from build123d import *

# Parameters (mm, degrees)
CROQUIS2_W              = 500
CROQUIS2_H              = 350
SALIENTE_EXTRUIR1_DEPTH = 50
CROQUIS3_W              = 125
CROQUIS3_H              = 87.5
SALIENTE_EXTRUIR2_DEPTH = 500


with BuildPart() as part:
    # Croquis2 → Saliente-Extruir1 (new body)
    with BuildSketch(Plane(origin=(0, 0, 0), x_dir=(1, 0, 0), z_dir=(0, 1, 0))):
        Rectangle(CROQUIS2_W, CROQUIS2_H)
    extrude(amount=SALIENTE_EXTRUIR1_DEPTH)

    # Croquis3 → Saliente-Extruir2 (add)
    with BuildSketch(Plane.XZ):
        with Locations((-187.5, 131.25)):
            Rectangle(CROQUIS3_W, CROQUIS3_H)
        with Locations((-187.5, -131.25)):
            Rectangle(CROQUIS3_W, CROQUIS3_H)
        with Locations((187.5, -131.25)):
            Rectangle(CROQUIS3_W, CROQUIS3_H)
        with Locations((187.5, 131.25)):
            Rectangle(CROQUIS3_W, CROQUIS3_H)
    extrude(amount=SALIENTE_EXTRUIR2_DEPTH)


solid = part.part
Could you check a few things on this model? Use its own coordinates, in mm. A direction names the side the tool comes from. Round coordinates to 2 decimals unless told otherwise and drop trailing zeros. Write each loop counter-clockwise with the first axis right and the second up, starting at its lowest first coordinate (ties: lowest second). Pieces come first, ordered by that corner, then holes. Notation, with made-up numbers: (81.5, 75.25) - (104.5, 75.25) arc R18 cw to (104.5, 91.25) - close; hole circle Ø9 at (28.25, -24.75). An arc over 180 degrees is marked (long way). Use a Markdown table: item, result.
Q1. Please list where these lines run through material, in increasing order: L1, parallel to Z at x = -138, y = -269; L2, parallel to X at y = -158, z = 119.5; L3, parallel to Y at x = -213, z = 63.
Output values:
| item | result |
|---|---|
| L1 | -175 to -87.5, 87.5 to 175 |
| L2 | -250 to -125, 125 to 250 |
| L3 | 0 to 50 |
Q2. I want a section at A-A (y = -410.5). List the corners of the cut face in (x, z) for me, plus the area to 4 significant figures.
Output values:
| item | result |
|---|---|
| outline | (-250, -175) - (-125, -175) - (-125, -87.5) - (-250, -87.5) - close; (-250, 87.5) - (-125, 87.5) - (-125, 175) - (-250, 175) - close; (125, -175) - (250, -175) - (250, -87.5) - (125, -87.5) - close; (125, 87.5) - (250, 87.5) - (250, 175) - (125, 175) - close |
| area | 43,750 mm2 |
Q3. Thinking about a two-plate mould opening in X: for faces 1 (the flat face through (-188, -246, -87.5)), 2 (the flat face through (250, -229, -114)), 3 (the flat face through (-125, -246, -132)), which applies, released by +X, released by -X, zero draft, split by the parting line, or undercut?
Output values:
| item | result |
|---|---|
| face 1 | zero draft |
| face 2 | released by +X |
| face 3 | undercut |
Q4. I want a section at B-B (x = -192). List the corners of the cut face in (y, z) for me.
Output values:
| item | result |
|---|---|
| outline | (-500, -175) - (50, -175) - (50, 175) - (-500, 175) - (-500, 87.5) - (0, 87.5) - (0, -87.5) - (-500, -87.5) - close |
Q5. I want a section at C-C (z = -152.5). List the corners of the cut face in (x, y) for me.
Output values:
| item | result |
|---|---|
| outline | (-250, -500) - (-125, -500) - (-125, 0) - (125, 0) - (125, -500) - (250, -500) - (250, 50) - (-250, 50) - close |
Q6. I want a section at D-D (z = -25.5). List the corners of the cut face in (x, y) for me.
Output values:
| item | result |
|---|---|
| outline | (-250, 0) - (250, 0) - (250, 50) - (-250, 50) - close |
Q7. For faces 4 (the flat face through (125, -246, -132)), 5 (the flat face through (-188, -500, 132)), 6 (the flat face through (187, -246, -87.5)), which set-ups out of +Z, -Z, +X, -X, +Y, -Y let a thin tool reach every point of the face, with its end or its side?
Output values:
| item | result |
|---|---|
| face 4 | +Z, -Z, -Y |
| face 5 | +Z, -Z, +X, -X, -Y |
| face 6 | +X, -X, -Y |
Q8. For pin 1 (10 mm diameter, centred on x = 154, z = 19, fed in from -Y), with a flat end and sliding along its axis, tell me the tip position at first contact or that it passes through.
Output values:
| item | result |
|---|---|
| pin 1 | y = 0 |
